Source: CAD feature listing. Evaluate the final solid. Frame: model axes, mm. Face numbers are marked on the shaded views. A direction names the side the tool comes from. Give positions to 0.01 mm unless a question says otherwise; leave off trailing zeros. Loops run counter-clockwise (first coordinate to the right, second up) from the corner with the lowest first, then second, coordinate; pieces in that order, holes last. Notation, with made-up numbers: M 48,65 L 83,65 A20 cw 83,84 Z; hole C 35,61.5 d3. An arc over 180 degrees is marked long. Answer in a Markdown table with one row per item.
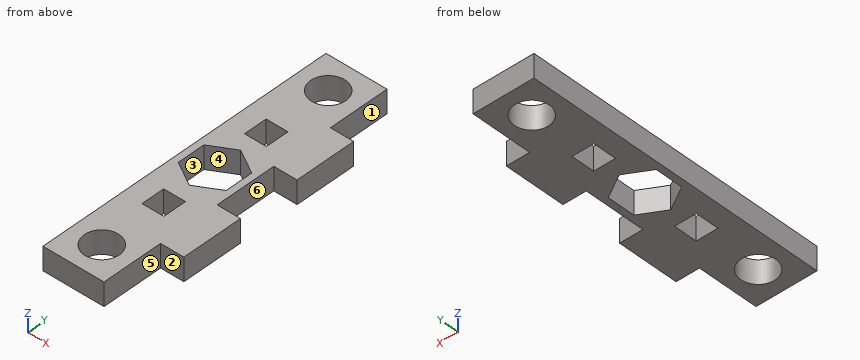
```python
from build123d import *

# Parameters (mm, degrees)
MODEL_R             = 4
MODEL_W             = 5
MODEL_H             = 5.35
BOSS_EXTRUDE1_DEPTH = 5.35


with BuildPart() as part:
    # Model → Boss-Extrude1 (new body)
    with BuildSketch(Plane.XY):
        Polygon((0, 0), (14, 0), (14, 14), (19.35, 14), (19.35, 28), (14, 28), (14, 42), (19.35, 42), (19.35, 56), (14, 56), (14, 70), (0, 70), align=None)
        with Locations((7, 63)):
            Circle(MODEL_R, mode=Mode.SUBTRACT)
        with Locations(Location((7, 7, 0), (0, 0, 180))):
            Circle(MODEL_R, mode=Mode.SUBTRACT)
        with Locations((7, 47.675)):
            Rectangle(MODEL_W, MODEL_H, mode=Mode.SUBTRACT)
        with Locations((7, 22.325)):
            Rectangle(MODEL_W, MODEL_H, mode=Mode.SUBTRACT)
        Polygon((1.500738686, 38.175), (1.500738686, 31.825), (7, 28.65), (12.499261314, 31.825), (12.499261314, 38.175), (7, 41.35), align=None, mode=Mode.SUBTRACT)
    extrude(amount=BOSS_EXTRUDE1_DEPTH)


solid = part.part
```
1) Material intervals for L1, parallel to Y at x = 7, z = 3; L2, parallel to Y at x = 17.25, z = 1.95; L3, parallel to Y at x = 9.75, z = 4.75, sorted ascending.
Reply:
| item | result |
|---|---|
| L1 | y = 0 to 3, 11 to 19.65, 25 to 28.65, 41.35 to 45, 50.35 to 59, 67 to 70 |
| L2 | y = 14 to 28, 42 to 56 |
| L3 | y = 0 to 4.1, 9.9 to 30.24, 39.76 to 60.1, 65.9 to 70 |
2) Section B-B, the plane x = 17. Return loops of the section in (y, z).
Reply:
| item | result |
|---|---|
| outline | M 14,0 L 28,0 L 28,5.35 L 14,5.35 Z; M 42,0 L 56,0 L 56,5.35 L 42,5.35 Z |
3) Section C-C, the plane z = 3.4. Return loops of the section in (x, y) (3 decimals).
Reply:
| item | result |
|---|---|
| outline | M 0,0 L 14,0 L 14,14 L 19.35,14 L 19.35,28 L 14,28 L 14,42 L 19.35,42 L 19.35,56 L 14,56 L 14,70 L 0,70 Z; hole M 1.501,31.825 L 7,28.65 L 12.499,31.825 L 12.499,38.175 L 7,41.35 L 1.501,38.175 Z; hole C 7,7 d8; hole C 7,63 d8; hole M 4.5,19.65 L 9.5,19.65 L 9.5,25 L 4.5,25 Z; hole M 4.5,45 L 9.5,45 L 9.5,50.35 L 4.5,50.35 Z |
4) Section D-D, the plane x = 8.5. Return loops of the section in (y, z), then the cut area to 3 significant figures.
Reply:
| item | result |
|---|---|
| outline | M 0,0 L 3.29,0 L 3.29,5.35 L 0,5.35 Z; M 10.71,0 L 19.65,0 L 19.65,5.35 L 10.71,5.35 Z; M 25,0 L 29.52,0 L 29.52,5.35 L 25,5.35 Z; M 40.48,0 L 45,0 L 45,5.35 L 40.48,5.35 Z; M 50.35,0 L 59.29,0 L 59.29,5.35 L 50.35,5.35 Z; M 66.71,0 L 70,0 L 70,5.35 L 66.71,5.35 Z |
| area | 179 mm² |
5) Set-up query: the marked faces 4, 5 and 6. Return all of +Z, -Z, +X, -X, +Y, -Y with unobstructed straight access to the full face (end or side cutting, diameter ignored); none if empty.
Reply:
| item | result |
|---|---|
| face 4 | +Z, -Z |
| face 5 | +Z, -Z, +X, -Y |
| face 6 | +Z, -Z, +X |
6) Pin query (flat end, axial travel): pin 1 Ø1.6 at (x, z) = (16, 2) entering from -Y; pin 2 Ø1 at (y, z) = (49, 4.5) entering from -X; pin 3 Ø2.5 at (y, z) = (60, 3) entering from +X; pin 4 Ø1.6 at (x, z) = (16.5, 2.5) entering from +Y. Return the tip coordinate at first contact, or that it passes through.
Reply:
| item | result |
|---|---|
| pin 1 | stops at y = 14 |
| pin 2 | stops at x = 0 |
| pin 3 | stops at x = 14 |
| pin 4 | stops at y = 56 |
7) Section A-A, the plane y = 63. Return loops of the section in (x, z).
Reply:
| item | result |
|---|---|
| outline | M 0,0 L 3,0 L 3,5.35 L 0,5.35 Z; M 11,0 L 14,0 L 14,5.35 L 11,5.35 Z |
8) Pull-direction query (Y, two-part tool) for the marked faces 1, 2 and 3; classes: released by +Y, released by -Y, zero draft, split by the parting line, or undercut.
Reply:
| item | result |
|---|---|
| face 1 | zero draft |
| face 2 | released by -Y |
| face 3 | undercut |
